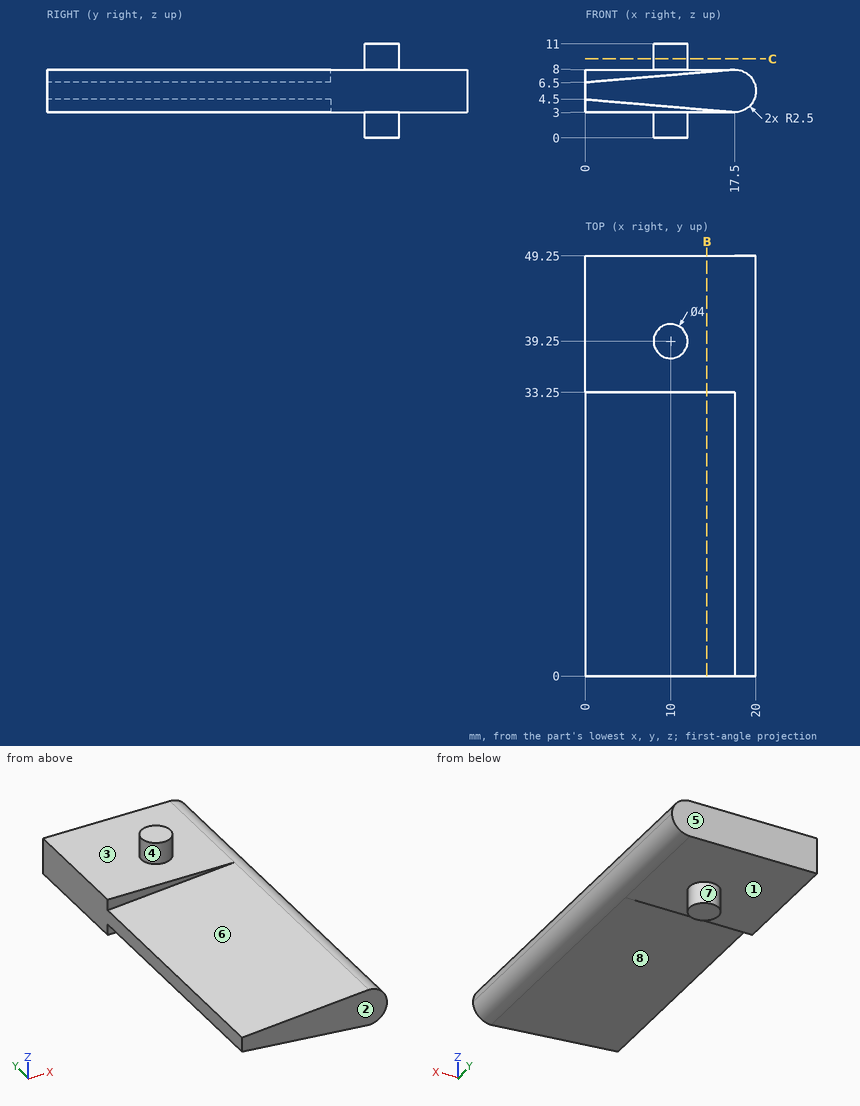
Here's the drawing with two shaded views (mm, measured from the low corner). I have some questions. A direction names the side the tool comes from. Coordinates: 2 decimals unless noted, no trailing zeros. Loops run counter-clockwise (first coordinate to the right, second up) from the corner with the lowest first, then second, coordinate; pieces in that order, holes last. Notation, with made-up numbers: M 8.5,5.5 L 24.5,5.5 A22 cw 24.5,42.5 Z; hole C 78,-2 d4. An arc over 180 degrees is marked long. Return JSON: item names as keys, results as strings. Group by question number.
Item 1: Imagine slicing it at B-B (x = 14.25). Please give me the cut outline in (y, z), and give its area (3 significant figures).
Item 2: Thinking about a two-plate mould opening in Z: for the marked faces 1, 2 and 3, which applies, released by +Z, released by -Z, zero draft, split by the parting line, or undercut?
Item 3: On a 3-axis mill with a long thin cutter (end or side, diameter ignored), from which of +Z, -Z, +X, -X, +Y, -Y can I reach the whole of each face in a straight line? I mean the marked faces 4, 5, 6, 7 and 8. Say none if no direction works.
Item 4: I'm going to push flat-ended pins straight in: pin 1 Ø9 at (x, y) = (12, 12.5) entering from -Z; pin 2 Ø3 at (x, y) = (11.5, 10) entering from +Z; pin 3 Ø1 at (x, y) = (7, 30.5) entering from +Z. Where does each tip first touch, or does it pass through?
Item 5: Imagine slicing it at C-C (z = 9.25). Please give me the cut outline in (x, y).
Item 6: If I drill on L1, parallel to Y at x = 5.25, z = 3.5; L2, parallel to Z at x = 16.75, y = 46; L3, parallel to Z at x = 2.25, y = 31, over which ranges is the centre line in solid material (lowest first)? Write a range as from..to.
Verdict:
{
 "1": {"outline": "M 0,3.28 L 33.25,3.28 L 33.25,3 L 49.25,3 L 49.25,8 L 33.25,8 L 33.25,7.72 L 0,7.72 Z", "area": "228 mm^2"},
 "2": {"face 1": "released by -Z", "face 2": "zero draft", "face 3": "released by +Z"},
 "3": {"face 4": "+Z", "face 5": "+Z, -Z, +X, -X, +Y", "face 6": "+Z, -X, -Y", "face 7": "-Z", "face 8": "-Z, -X, -Y"},
 "4": {"pin 1": "stops at z = 3.09", "pin 2": "stops at z = 7.61", "pin 3": "stops at z = 7.14"},
 "5": {"outline": "C 10,39.25 d4"},
 "6": {"L1": "y = 33.25..49.25", "L2": "z = 3..8", "L3": "z = 4.31..6.69"}
}
